Could you check a few things on this model? Use its own coordinates, in mm. A direction names the side the tool comes from. Round coordinates to 2 decimals unless told otherwise and drop trailing zeros. Order: outer loops, then holes, each group sorted by start corner. A loop starts at its lowest first (then second) coordinate and runs counter-clockwise, first axis right, second up. Notation, with made-up numbers: (87, 40.25) - (100, 40.25) arc R17 ccw to (100, 60.25) - close; hole circle Ø6 at (-32, 80). An arc over 180 degrees is marked (long way). Return JSON: item names as keys, results as strings. Group by question number.
Autodesk Fusion 360 part; units mm, degrees
sketch "Esboço1" plane through (0, 0, 0) normal (0, 0, 1) x (1, 0, 0)
  circle A0 centre (0, 0) radius 240
  line L0 (48, -48) -> (-48, -48)
  line L1 (-48, -48) -> (-48, 48)
  line L2 (-48, 48) -> (48, 48)
  line L3 (48, 48) -> (48, -48)
  line L4 (48, -48) -> (-48, 48) construction
  line L5 (-48, -48) -> (48, 48) construction
  circle A1 centre (-48, 48) radius 5
  circle A2 centre (-48, -48) radius 5
  circle A3 centre (48, 48) radius 5
  circle A4 centre (48, -48) radius 5
  line L6 (105, -110) -> (105, -170)
  line L7 (90, -125) -> (90, -155)
  line L8 (120, -125) -> (120, -155)
  arc A5 (120, -125) -> (90, -125) centre (105, -125) ccw
  arc A6 (90, -155) -> (120, -155) centre (105, -155) ccw
  circle A7 centre (148, -148) radius 5
  line L9 (-125, 204.878) -> (125, 204.878)
  circle A8 centre (0, 311.043) radius 164
  circle A9 centre (107.5, 130.5) radius 5
  line L10 (-40, 115) -> (40, 115)
  line L11 (-40, 115) -> (-40, 151.9958)
  line L12 (40, 115) -> (40, 151.9958)
  line L13 (0, 1.75) -> (0, 22.5)
  line L14 (-120, -125) -> (-120, -155)
  arc A10 (-90, -125) -> (-120, -125) centre (-105, -125) ccw
  line L15 (-90, -125) -> (-90, -155)
  arc A11 (-120, -155) -> (-90, -155) centre (-105, -155) ccw
  circle A12 centre (-148, -148) radius 5
  circle A13 centre (-107.5, 130.5) radius 5
  line L16 (-45, -185) -> (45, -185)
  line L17 (45, -185) -> (45, -240)
  line L18 (45, -240) -> (-45, -240)
  line L19 (-45, -240) -> (-45, -185)
  line L20 (0, -185) -> (0, -175)
  line L21 (-37.5, -175) -> (37.5, -175)
  circle A14 centre (-37.5, -175) radius 2.5
  circle A15 centre (37.5, -175) radius 2.5
  circle A16 centre (37.5, -115) radius 2.5
  circle A17 centre (37.5, -55) radius 2.5
  circle A18 centre (-37.5, -115) radius 2.5
  circle A19 centre (-37.5, -55) radius 2.5
  circle A20 centre (132.8044, 119.976) radius 2.5
  line L22 (230.3461, 81.0289) -> (182.7147, 53.5289)
  line L23 (182.7147, 53.5289) -> (137.7147, 131.4711)
  line L24 (137.7147, 131.4711) -> (185.3461, 158.9711)
  circle A21 centre (80.8429, 89.976) radius 2.5
  circle A22 centre (170.3044, 55.024) radius 2.5
  circle A23 centre (118.3429, 25.024) radius 2.5
  circle A24 centre (66.3814, -4.976) radius 2.5
  circle A25 centre (28.8814, 59.976) radius 2.5
  circle A26 centre (-170.3044, 55.024) radius 2.5
  line L25 (-185.3461, 158.9711) -> (-137.7147, 131.4711)
  line L26 (-137.7147, 131.4711) -> (-182.7147, 53.5289)
  line L27 (-182.7147, 53.5289) -> (-230.3461, 81.0289)
  circle A27 centre (-118.3429, 25.024) radius 2.5
  circle A28 centre (-132.8044, 119.976) radius 2.5
  circle A29 centre (-80.8429, 89.976) radius 2.5
  circle A30 centre (-28.8814, 59.976) radius 2.5
  circle A31 centre (-66.3814, -4.976) radius 2.5
  line L28 (0, -185) -> (0, -160)
  line L29 (-22.5, -160) -> (22.5, -160)
  circle A32 centre (-22.5, -160) radius 5
  circle A33 centre (22.5, -160) radius 5
  circle A34 centre (-22.5, -111) radius 5
  circle A35 centre (22.5, -111) radius 5
  circle A36 centre (149.8141, 60.5144) radius 5
  circle A37 centre (107.3788, 36.0144) radius 5
  circle A38 centre (84.8788, 74.9856) radius 5
  circle A39 centre (127.3141, 99.4856) radius 5
  circle A40 centre (-127.3141, 99.4856) radius 5
  circle A41 centre (-84.8788, 74.9856) radius 5
  circle A42 centre (-107.3788, 36.0144) radius 5
  circle A43 centre (-149.8141, 60.5144) radius 5
  line L30 (-17.902, -79) -> (18.098, -79)
  circle A44 centre (-17.902, -79) radius 1.75
  circle A45 centre (18.098, -79) radius 1.75
  line L31 (0, 311.043) -> (0, 115)
  circle A46 centre (-17.902, 67) radius 1.75
  circle A47 centre (18.098, 67) radius 1.75
  point P0 (105, -110)
  point P1 (0, 115)
  point P2 (0, -240)
  point P3 (-45, -235.7435)
  point P4 (-181.6599, 156.8429)
  point P5 (181.6599, 156.8429)
  point P6 (0.098, -79)
  dimension "d1" = 480
  dimension "d2" = 96
  dimension "d3" = 96
  dimension "d4" = 10
  dimension "d5" = 10
  dimension "d6" = 10
  dimension "d7" = 10
  dimension "d8" = 110
  dimension "d9" = 105
  dimension "d10" = 30
  dimension "d11" = 60
  dimension "d12" = 30
  dimension "d13" = 10
  dimension "d14" = 148
  dimension "d15" = 148
  dimension "d16" = 250
  dimension "d17" = 328
  dimension "d18" = 10
  dimension "d19" = 130.5
  dimension "d20" = 107.5
  dimension "d21" = 115
  dimension "d22" = 80
  dimension "d25" = 90
  dimension "d26" = 55
  dimension "d27" = 10
  dimension "d28" = 75
  dimension "d29" = 5
  dimension "d30" = 5
  dimension "d33" = 1
  dimension "d34" = 60
  dimension "d36" = 360
  dimension "d37" = 25
  dimension "d38" = 45
  dimension "d39" = 10
  dimension "d40" = 10
  dimension "d43" = 0
  dimension "d44" = 49
  dimension "d45" = 36
  dimension "d46" = 3.5
  dimension "d47" = 3.5
  dimension "d51" = 0
  dimension "d52" = 146
  dimension "d53" = 32
extrude "Extrusão1" add sketch "Esboço1" along normal blind 3 contours A0 A8 L10 L11 L12 L16 L17 L19 L22 L23 L24 L25 L26 L27 | A8 L10 L12 L31 | A8 L10 L11 L31 | L0 L1 L2 L3 A1 A2 A3 A4
equation "d12 = d10"
equation "d17 = ( 164 * 2 ) * 1 mm"
1) Will these pins go through, and if not, where does the flat tip stop? pin 1 (1.5 mm diameter, centred on y = -184.5, z = 2, fed in from -X); pin 2 (3 mm diameter, centred on x = -78, y = 104, fed in from -Z); pin 3 (4.5 mm diameter, centred on x = -118.34, y = 25.02, fed in from +Z); pin 4 (1.5 mm diameter, centred on x = -159, z = 1.5, fed in from -Y).
2) We'd pull the mould along Y, two halves only. Please class faces 1 (the cylindrical face through (1.99, 147.055, 1.479)), 2 (the cylindrical face through (-206.39, -122.49, 1.48)), 3 (the cylindrical face through (122.32, 99.27, 1.48)), 4 (the flat face through (-3, -12, 3)): +Y half, -Y half, draft (parallel to the pull), parting line (faces both ways), or undercut.
3) For faces 5 (the flat face through (-3, -12, 0)), 6 (the cylindrical face through (105, -170, 1)), 7 (the flat face through (204.99, 66.39, 1.48)), which set-ups out of +Z, -Z, +X, -X, +Y, -Y let a thin tool reach every point of the face, with its end or its side?
4) I want a section at C-C, the plane x = 3. List the corners of the cut face in (y, z) for me, plus the area to 3 significant figures.
5) I want a section at B-B, the plane y = -72. List the corners of the cut face in (x, z) for me.
6) I want a section at A-A, the plane z = 1.65. Give the number of separate pieces and of enclosed holes in the cut face, plus the area to 3 significant figures.
7) If I drill on line 1 along X through (y, z) = (-48, 2.3); line 2 along Y through (x, z) = (22.5, 2.05); line 3 along X through (y, z) = (90, 2.55), over which ranges is the centre line in solid material (lowest first)? Write a range as from..to.
Outcome:
{
 "1": {"pin 1": "x = -154.39", "pin 2": "z = 0", "pin 3": "through", "pin 4": "y = -180.44"},
 "2": {"face 1": "+Y half", "face 2": "parting line", "face 3": "undercut", "face 4": "draft"},
 "3": {"face 5": "-Z, +X, -X, +Y, -Y", "face 6": "+Z, -Z", "face 7": "+Z, -Z, +Y"},
 "4": {"outline": "(-185, 0) - (147.07, 0) - (147.07, 3) - (-185, 3) - close", "area": "996 mm^2"},
 "5": {"outline": "(-228.95, 0) - (228.95, 0) - (228.95, 3) - (-228.95, 3) - close"},
 "6": {"separate pieces": "1", "enclosed holes": "44", "area": "145,000 mm^2"},
 "7": {"line 1": "-235.15..-53, -43..43, 53..235.15", "line 2": "-185..-165, -155..-116, -106..148.59", "line 3": "-161.66..-83.34, -78.34..78.34, 83.34..161.66"}
}
